from build123d import *

# Parameters (mm, degrees)
SKETCH1_R             = 0.6
BOSS_EXTRUDE1_DEPTH   = 3
BOSS_EXTRUDE1_2_DEPTH = 3
BOSS_EXTRUDE1_3_DEPTH = 3
BOSS_EXTRUDE1_4_DEPTH = 3
BOSS_EXTRUDE2_DEPTH   = 1.3
BOSS_EXTRUDE3_DEPTH   = 3
CIRPATTERN1_COUNT     = 4


# Read off the part's stored shape, not the designer's step: M2 Clearance Hole1
with BuildPart() as part:
    # Sketch1 → Boss-Extrude1 (new body)
    with BuildSketch(Plane(origin=(0, 0, 0), x_dir=(0, 1, 0), z_dir=(0, 0, 1))):
        with BuildLine():
            Line((-1.5, 7.348469228), (-1.5, 24.954959427))
            ThreePointArc((-1.5, 24.954959427), (-17.67766953, 17.67766953), (-24.954959427, 1.5))
            Line((-24.954959427, 1.5), (-7.348469228, 1.5))
            ThreePointArc((-7.348469228, 1.5), (-6.756656365, 3.255394717), (-5.752639047, 4.812187028))
            Line((-5.752639047, 4.812187028), (-7.166852609, 6.226400591))
            Line((-7.166852609, 6.226400591), (-6.226400591, 7.166852609))
            Line((-6.226400591, 7.166852609), (-4.812187028, 5.752639047))
            ThreePointArc((-4.812187028, 5.752639047), (-3.255394717, 6.756656365), (-1.5, 7.348469228))
        make_face()
        with Locations(Location((-12.375, 12.375, 0), (0, 0, 270))):
            Circle(SKETCH1_R, mode=Mode.SUBTRACT)
    extrude(amount=BOSS_EXTRUDE1_DEPTH)

    # Sketch1<9> → Boss-Extrude2 (add)
    with BuildSketch(Plane(origin=(0, 0, 0), x_dir=(0, 1, 0), z_dir=(0, 0, 1))):
        with BuildLine():
            Line((1.5, 7.348469228), (1.5, 24.954959427))
            ThreePointArc((1.5, 24.954959427), (0, 25), (-1.5, 24.954959427))
            Line((-1.5, 24.954959427), (-1.5, 7.348469228))
            ThreePointArc((-1.5, 7.348469228), (0, 7.5), (1.5, 7.348469228))
        make_face()
        with BuildLine():
            ThreePointArc((-24.954959427, 1.5), (-25, 0), (-24.954959427, -1.5))
            Line((-24.954959427, -1.5), (-7.348469228, -1.5))
            ThreePointArc((-7.348469228, -1.5), (-7.5, 0), (-7.348469228, 1.5))
            Line((-7.348469228, 1.5), (-24.954959427, 1.5))
        make_face()
        with BuildLine():
            ThreePointArc((24.954959427, -1.5), (25, 0), (24.954959427, 1.5))
            Line((24.954959427, 1.5), (7.348469228, 1.5))
            ThreePointArc((7.348469228, 1.5), (7.5, 0), (7.348469228, -1.5))
            Line((7.348469228, -1.5), (24.954959427, -1.5))
        make_face()
        with BuildLine():
            ThreePointArc((-1.5, -24.954959427), (0, -25), (1.5, -24.954959427))
            Line((1.5, -24.954959427), (1.5, -7.348469228))
            ThreePointArc((1.5, -7.348469228), (0, -7.5), (-1.5, -7.348469228))
            Line((-1.5, -7.348469228), (-1.5, -24.954959427))
        make_face()
    extrude(amount=BOSS_EXTRUDE2_DEPTH)


with BuildPart() as body_2:
    # Sketch1 → Boss-Extrude1 2 (new body)
    with BuildSketch(Plane(origin=(0, 0, 0), x_dir=(0, 1, 0), z_dir=(0, 0, 1))):
        with BuildLine():
            Line((1.5, 24.954959427), (1.5, 7.348469228))
            ThreePointArc((1.5, 7.348469228), (3.255394717, 6.756656365), (4.812187028, 5.752639047))
            Line((4.812187028, 5.752639047), (6.226400591, 7.166852609))
            Line((6.226400591, 7.166852609), (7.166852609, 6.226400591))
            Line((7.166852609, 6.226400591), (5.752639047, 4.812187028))
            ThreePointArc((5.752639047, 4.812187028), (6.756656365, 3.255394717), (7.348469228, 1.5))
            Line((7.348469228, 1.5), (24.954959427, 1.5))
            ThreePointArc((24.954959427, 1.5), (17.67766953, 17.67766953), (1.5, 24.954959427))
        make_face()
        with Locations(Location((12.375, 12.375, 0), (0, 0, 270))):
            Circle(SKETCH1_R, mode=Mode.SUBTRACT)
    extrude(amount=BOSS_EXTRUDE1_2_DEPTH)

    # M2 Clearance Hole1 4 outline → M2 Clearance Hole1 4 (revolve, cut)
    with BuildSketch(Plane(origin=(-8.485, 8.485, 0), x_dir=(1, 0, 0), z_dir=(0, -1, 0))):
        Polygon((0, 0), (1.2, 0), (1.2, 2.975), (1.225, 3), (0, 3), align=None)
    revolve(axis=Axis((-8.485, 8.485, 0), (0, 0, 1)), mode=Mode.SUBTRACT)



with BuildPart() as body_3:
    # Sketch1 → Boss-Extrude1 3 (new body)
    with BuildSketch(Plane(origin=(0, 0, 0), x_dir=(0, 1, 0), z_dir=(0, 0, 1))):
        with BuildLine():
            Line((-7.348469228, -1.5), (-24.954959427, -1.5))
            ThreePointArc((-24.954959427, -1.5), (-17.67766953, -17.67766953), (-1.5, -24.954959427))
            Line((-1.5, -24.954959427), (-1.5, -7.348469228))
            ThreePointArc((-1.5, -7.348469228), (-3.255394717, -6.756656365), (-4.812187028, -5.752639047))
            Line((-4.812187028, -5.752639047), (-6.226400591, -7.166852609))
            Line((-6.226400591, -7.166852609), (-7.166852609, -6.226400591))
            Line((-7.166852609, -6.226400591), (-5.752639047, -4.812187028))
            ThreePointArc((-5.752639047, -4.812187028), (-6.756656365, -3.255394717), (-7.348469228, -1.5))
        make_face()
        with Locations(Location((-12.375, -12.375, 0), (0, 0, 270))):
            Circle(SKETCH1_R, mode=Mode.SUBTRACT)
    extrude(amount=BOSS_EXTRUDE1_3_DEPTH)

    # M2 Clearance Hole1 2 outline → M2 Clearance Hole1 2 (revolve, cut)
    with BuildSketch(Plane(origin=(8.485, -8.485, 0), x_dir=(1, 0, 0), z_dir=(0, -1, 0))):
        Polygon((0, 0), (1.2, 0), (1.2, 2.975), (1.225, 3), (0, 3), align=None)
    revolve(axis=Axis((8.485, -8.485, 0), (0, 0, 1)), mode=Mode.SUBTRACT)


with BuildPart() as body_4:
    # Sketch1 → Boss-Extrude1 4 (new body)
    with BuildSketch(Plane(origin=(0, 0, 0), x_dir=(0, 1, 0), z_dir=(0, 0, 1))):
        with BuildLine():
            Line((24.954959427, -1.5), (7.348469228, -1.5))
            ThreePointArc((7.348469228, -1.5), (6.756656365, -3.255394717), (5.752639047, -4.812187028))
            Line((5.752639047, -4.812187028), (7.166852609, -6.226400591))
            Line((7.166852609, -6.226400591), (6.226400591, -7.166852609))
            Line((6.226400591, -7.166852609), (4.812187028, -5.752639047))
            ThreePointArc((4.812187028, -5.752639047), (3.255394717, -6.756656365), (1.5, -7.348469228))
            Line((1.5, -7.348469228), (1.5, -24.954959427))
            ThreePointArc((1.5, -24.954959427), (17.67766953, -17.67766953), (24.954959427, -1.5))
        make_face()
        with Locations(Location((12.375, -12.375, 0), (0, 0, 270))):
            Circle(SKETCH1_R, mode=Mode.SUBTRACT)
    extrude(amount=BOSS_EXTRUDE1_4_DEPTH)

    # M2 Clearance Hole1 outline → M2 Clearance Hole1 (revolve, cut)
    with BuildSketch(Plane(origin=(8.485, 8.485, 0), x_dir=(1, 0, 0), z_dir=(0, -1, 0))):
        Polygon((0, 0), (1.2, 0), (1.2, 2.975), (1.225, 3), (0, 3), align=None)
    revolve(axis=Axis((8.485, 8.485, 0), (0, 0, 1)), mode=Mode.SUBTRACT)


with BuildPart() as boss_extrude2_piece_1:
    # of the separate pieces the step leaves, piece 1, a body of its own (boss_extrude2_pieces)
    add(part.part.solids().sort_by_distance((-24.954959427, -1.5, 1.3))[0])

    # M2 Clearance Hole1 3 outline → M2 Clearance Hole1 3 (revolve, cut)
    with BuildSketch(Plane(origin=(-8.485, -8.485, 0), x_dir=(1, 0, 0), z_dir=(0, -1, 0))):
        Polygon((0, 0), (1.2, 0), (1.2, 2.975), (1.225, 3), (0, 3), align=None)
    revolve(axis=Axis((-8.485, -8.485, 0), (0, 0, 1)), mode=Mode.SUBTRACT)


with BuildPart() as boss_extrude2_piece_2:
    # of the separate pieces the step leaves, piece 2, a body of its own (boss_extrude2_pieces)
    add(part.part.solids().sort_by_distance((-1.5, 7.348469228, 0))[0])


with BuildPart() as boss_extrude2_piece_3:
    # of the separate pieces the step leaves, piece 3, a body of its own (boss_extrude2_pieces)
    add(part.part.solids().sort_by_distance((24.954959427, -1.5, 0))[0])


with BuildPart() as body_2_1:
    add(body_2.part)

    add(body_3.part)  # Boss-Extrude3 merges body 3

    add(body_4.part)  # Boss-Extrude3 merges body 4

    add(boss_extrude2_piece_1.part)  # Boss-Extrude3 merges Boss-Extrude2 piece 1

    add(boss_extrude2_piece_2.part)  # Boss-Extrude3 merges Boss-Extrude2 piece 2

    add(boss_extrude2_piece_3.part)  # Boss-Extrude3 merges Boss-Extrude2 piece 3
    # Sketch1<10> → Boss-Extrude3 (add)
    with BuildSketch(Plane(origin=(0, 0, 0), x_dir=(0, 1, 0), z_dir=(0, 0, 1))):
        with BuildLine():
            Line((-1.5, -7.348469228), (-1.5, -8.7))
            Line((-1.5, -8.7), (1.5, -8.7))
            Line((1.5, -8.7), (1.5, -7.348469228))
            ThreePointArc((1.5, -7.348469228), (0, -7.5), (-1.5, -7.348469228))
        make_face()
        with BuildLine():
            Line((-7.348469228, 1.5), (-8.7, 1.5))
            Line((-8.7, 1.5), (-8.7, -1.5))
            Line((-8.7, -1.5), (-7.348469228, -1.5))
            ThreePointArc((-7.348469228, -1.5), (-7.5, 0), (-7.348469228, 1.5))
        make_face()
        with BuildLine():
            Line((1.5, 8.7), (-1.5, 8.7))
            Line((-1.5, 8.7), (-1.5, 7.348469228))
            ThreePointArc((-1.5, 7.348469228), (0, 7.5), (1.5, 7.348469228))
            Line((1.5, 7.348469228), (1.5, 8.7))
        make_face()
        with BuildLine():
            Line((8.7, -1.5), (8.7, 1.5))
            Line((8.7, 1.5), (7.348469228, 1.5))
            ThreePointArc((7.348469228, 1.5), (7.5, 0), (7.348469228, -1.5))
            Line((7.348469228, -1.5), (8.7, -1.5))
        make_face()
    extrude(amount=BOSS_EXTRUDE3_DEPTH)

    # Sketch8 → CBORE for M2 SHCS1 (revolve, cut)
    with BuildSketch(Plane(origin=(16.584366049, 16.584366049, 3), x_dir=(0, -1, 0), z_dir=(1, 0, 0))):
        Polygon((0, 0), (0, 3), (1.2, 3), (1.2, 2), (2.2, 2), (2.2, 0.025), (2.225, 0), align=None)
    cbore_for_m2_shcs1 = revolve(axis=Axis((16.584366049, 16.584366049, 9.35), (0, 0, -1)), mode=Mode.SUBTRACT)

    # CirPattern1: CBORE for M2 SHCS1 ×4 about axis
    cirpattern1_axis = Axis((0, 0, 0), (0, 0, 1))
    for i in range(1, CIRPATTERN1_COUNT):
        add(cbore_for_m2_shcs1.rotate(cirpattern1_axis, i * 360 / CIRPATTERN1_COUNT), mode=Mode.SUBTRACT)


solid = body_2_1.part
Can you work these out from the model? Positions are in its coordinate system, mm. A direction names the side the tool comes from. Coordinates: 2 decimals unless noted, no trailing zeros. Order: outer loops, then holes, each group sorted by start corner. A loop starts at its lowest first (then second) coordinate and runs counter-clockwise, first axis right, second up. Notation, with made-up numbers: M 67,67.25 L 119,67.25 A24 ccw 119,105.25 Z; hole C 84,52.5 d3. An arc over 180 degrees is marked long. Answer as CSV lines item,"result".
(1) Please list where these lines run through material, in increasing order: L1, parallel to X at y = -16.5, z = 0.95; L2, parallel to Y at x = 0, z = 0.75; L3, parallel to X at y = 8.5, z = 2.2.
Geometry check:
L1,"-18.78 to -17.78, -15.39 to 15.39, 17.78 to 18.78"
L2,"-25 to -7.5, 7.5 to 25"
L3,"-23.51 to -9.68, -7.29 to 7.29, 9.68 to 23.51"
(2) On a 3-axis mill with a long thin cutter (end or side, diameter ignored), from which of +Z, -Z, +X, -X, +Y, -Y can I reach the whole of each face in a straight line? I mean faces 1 (the flat face through (-17, 0, 1.3)), 2 (the flat face through (0, -17, 1.3)), 3 (the flat face through (1.5, 17, 2)), 4 (the flat face through (5.51, 6.45, 1.48)), 5 (the cylindrical face through (-14.98, 15.08, 2)). Say none if no direction works.
Geometry check:
face 1,"+Z, -X"
face 2,"+Z, -Y"
face 3,"+Z, +Y"
face 4,"+Z, -Z"
face 5,"+Z"
(3) I'm going to push flat-ended pins straight in: pin 1 (1.3 mm diameter, centred on x = 15.5, y = -16.5, fed in from +Z); pin 2 (0.5 mm diameter, centred on y = -17.5, z = 2.5, fed in from -X); pin 3 (0.8 mm diameter, centred on y = 13.5, z = 2, fed in from +X). Where does each tip first touch, or does it pass through?
Geometry check:
pin 1,"z = 1"
pin 2,"x = -14.72"
pin 3,"x = 21.29"
(4) Suppose I cut it at A-A on x = 0. Please give me the cut outline in (y, z).
Geometry check:
outline,"M -25,0 L -7.5,0 L -7.5,3 L -8.7,3 L -8.7,1.3 L -25,1.3 Z; M 7.5,0 L 25,0 L 25,1.3 L 8.7,1.3 L 8.7,3 L 7.5,3 Z"
(5) If we mould it in two halves opening along X, with no side actions, what happens to faces 6 (the flat face through (17, -1.5, 2)), 7 (the flat face through (0, -8.7, 2))? For each: released by +X, released by -X, zero draft, split by the parting line, or undercut.
Geometry check:
face 6,"zero draft"
face 7,"undercut"
(6) Suppose I cut it at C-C on x = 19.5. Please give me the cut outline in (y, z), plus the area to 3 significant figures.
Geometry check:
outline,"M -15.64,0 L 15.64,0 L 15.64,3 L 1.5,3 L 1.5,1.3 L -1.5,1.3 L -1.5,3 L -15.64,3 Z"
area,"88.8 mm^2"
(7) Suppose I cut it at D-D on z = 2. Count the separate pieces of the cut face and the enclosed holes in it, plus the area to 3 significant figures.
Geometry check:
separate pieces,"1"
enclosed holes,"9"
area,"1,500 mm^2"
(8) Suppose I cut it at B-B on y = -20. Please give me the cut outline in (x, z).
Geometry check:
outline,"M -15,0 L 15,0 L 15,3 L 1.5,3 L 1.5,1.3 L -1.5,1.3 L -1.5,3 L -15,3 Z"
